```python
from build123d import *

# Parameters (mm, degrees)
SKETCH1_R           = 15
BOSS_EXTRUDE1_DEPTH = 30


with BuildPart() as part:
    # Sketch1 → Boss-Extrude1 (new body)
    with BuildSketch(Plane.XY):
        with BuildLine():
            Line((30, 25), (30, 5))
            Line((30, 5), (60, 5))
            Line((60, 5), (60, -5))
            Line((60, -5), (-60, -5))
            Line((-60, -5), (-60, 5))
            Line((-60, 5), (-30, 5))
            Line((-30, 5), (-30, 25))
            ThreePointArc((-30, 25), (0, 55), (30, 25))
        make_face()
        with Locations((0, 25)):
            Circle(SKETCH1_R, mode=Mode.SUBTRACT)
    extrude(amount=BOSS_EXTRUDE1_DEPTH)


solid = part.part
```
Geometry check sheet. Reference: the model listing, model coordinates, mm. A direction names the side the tool comes from. Give positions to 0.01 mm unless a question says otherwise; leave off trailing zeros. Write each loop counter-clockwise with the first axis right and the second up, starting at its lowest first coordinate (ties: lowest second). Pieces come first, ordered by that corner, then holes. Notation, with made-up numbers: (-7.75, 52.25) -> (36.25, 52.25) arc R25 cw to (36.25, 87.25) -> close; hole circle Ø1 at (64.5, 44.5). An arc over 180 degrees is marked (long way). One line per question, with ' | ' between items.
Item 1: Depth check by flat-ended pin: pin 1 (9 mm diameter, centred on x = -39, z = 17.5, fed in from +Y); pin 2 (10 mm diameter, centred on y = 17, z = 8, fed in from -X); pin 3 (16 mm diameter, centred on y = 18, z = 19, fed in from +X); pin 4 (6 mm diameter, centred on x = -14.5, y = 42.5, fed in from -Z). Enter the tip coordinate at first touch or a pass-through.
Determined:
pin 1: y = 5 | pin 2: x = -30 | pin 3: x = 30 | pin 4: z = 0
Item 2: Access from +Z, -Z, +X, -X, +Y, -Y to the whole of each face (thin tool, end or side, straight path). Record for faces 1 (the flat face through (45, 5, 15)), 2 (the flat face through (-30, 15, 15)), 3 (the cylindrical face through (-0.66, 54.993, 14.79)).
Determined:
face 1: +Z, -Z, +X, +Y | face 2: +Z, -Z, -X, +Y | face 3: +Z, -Z, +Y
Item 3: Draft check along Y on faces 4 (the flat face through (-45, 5, 15)), 5 (the cylindrical face through (-3.252, 10.357, 14.79)), 6 (the flat face through (1, 5, 30)). Enter one of: released by +Y, released by -Y, zero draft, split by the parting line, or undercut.
Determined:
face 4: released by +Y | face 5: undercut | face 6: zero draft
Item 4: Sectioned sample at C-C, the plane y = 31.5. Record the boundary of the cut face in (x, z).
Determined:
outline: (-29.29, 0) -> (-13.52, 0) -> (-13.52, 30) -> (-29.29, 30) -> close; (13.52, 0) -> (29.29, 0) -> (29.29, 30) -> (13.52, 30) -> close
Item 5: Sectioned sample at A-A, the plane x = 0. Record the boundary of the cut face in (y, z).
Determined:
outline: (-5, 0) -> (10, 0) -> (10, 30) -> (-5, 30) -> close; (40, 0) -> (55, 0) -> (55, 30) -> (40, 30) -> close
Item 6: Scan lines: line 1 along Y through (x, z) = (0, 13.75); line 2 along Y through (x, z) = (49, 2.5); line 3 along Y through (x, z) = (3, 16). Record each from-to range of solid material in increasing order.
Determined:
line 1: -5 to 10, 40 to 55 | line 2: -5 to 5 | line 3: -5 to 10.3, 39.7 to 54.85
Item 7: Sectioned sample at D-D, the plane x = 46.5. Record the boundary of the cut face in (y, z).
Determined:
outline: (-5, 0) -> (5, 0) -> (5, 30) -> (-5, 30) -> close
Item 8: Sectioned sample at B-B, the plane z = 7. Record the boundary of the cut face in (x, y).
Determined:
outline: (-60, -5) -> (60, -5) -> (60, 5) -> (30, 5) -> (30, 25) arc R30 ccw to (-30, 25) -> (-30, 5) -> (-60, 5) -> close; hole circle Ø30 at (0, 25)
